from build123d import *

# Parameters (mm, degrees)
F0_W     = 203.2
F0_H     = 152.4
F1_DEPTH = 19.05
F2_SIZE  = 6.35
F4_D     = 25.4
F5_W     = 31.75
F5_H     = 31.75
F7_R     = 6.35
F8_SIZE  = 3.81


with BuildPart() as f1:
    # F0 (on Top) → F1 (new body)
    with BuildSketch(Plane.XY):
        Rectangle(F0_W, F0_H)
    extrude(amount=F1_DEPTH)

    # F2
    f2_edges = [f1.edges().sort_by_distance(p)[0] for p in [
        (0, -76.2, 19.05),
        (101.6, 0, 19.05),
        (-101.6, 0, 19.05),
        (0, 76.2, 19.05),
    ]]
    chamfer(f2_edges, length=F2_SIZE)

    # F4 (through all)
    with Locations(Plane.XY.offset(19.05)):
        with Locations((-69.85, 44.45), (69.85, 44.45), (69.85, -44.45), (-69.85, -44.45)):
            Hole(F4_D / 2)

    # F5 (on Front) → F6 (revolve)
    with BuildSketch(Plane.XZ):
        Polygon((0, 114.3), (0, 82.55), (31.75, 82.55), (44.45, 82.55), (44.45, 114.3), align=None)
        with Locations((15.875, 66.675)):
            Rectangle(F5_W, F5_H)
        Polygon((31.75, 50.8), (0, 50.8), (0, 19.05), (44.45, 19.05), (44.45, 50.8), align=None)
    revolve(axis=Axis((0, 0, 34.925), (0, 0, -1)))

    # F7
    f7_edges = [f1.edges().sort_by_distance(p)[0] for p in [
        (-44.45, 0, 114.3),
        (-44.45, 0, 19.05),
    ]]
    fillet(f7_edges, radius=F7_R)

    # F8
    f8_edges = [f1.edges().sort_by_distance(p)[0] for p in [
        (-44.45, 0, 50.8),
        (-44.45, 0, 82.55),
    ]]
    chamfer(f8_edges, length=F8_SIZE)


solid = f1.part
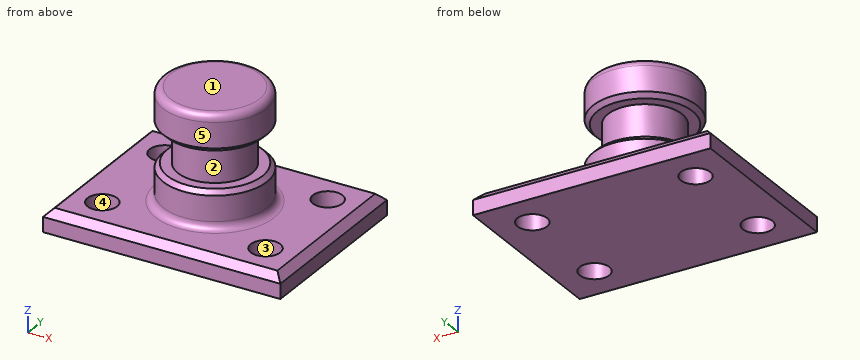
Input: part model. Units: mm. Frame: model coordinates. Face numbers are marked on the shaded views. A direction names the side the tool comes from. Give positions to 0.01 mm unless a question says otherwise; leave off trailing zeros. Loops run counter-clockwise (first coordinate to the right, second up) from the corner with the lowest first, then second, coordinate; pieces in that order, holes last. Notation, with made-up numbers: (7.5, -11) -> (33.5, -11) arc R11 cw to (33.5, 1) -> close; hole circle Ø10 at (77.25, 52.5). An arc over 180 degrees is marked (long way). Answer as a JSON object with one key per item and string values. Group by question number.
Item 1: Line query: probe 1 along X at (y, z) = (44, 10); probe 2 along Y at (x, z) = (-69, 10); probe 3 along Y at (x, z) = (64.5, 16.5). Output: solid intervals per line, ascending.
Item 2: Cut plane D-D, the plane z = 64.5. Return the cut outline in (x, y), and give its area (3 significant figures).
Item 3: Pull-direction query (Y, two-part tool) for the marked faces 1, 2 and 3; classes: released by +Y, released by -Y, zero draft, split by the parting line, or undercut.
Item 4: Pin query (flat end, axial travel): P1, Ø1, axis at x = 8, z = 78, coming from the -Y side; P2, Ø6, axis at x = 28, z = 87, coming from the -Y side; P3, Ø15, axis at x = -69.85, y = 44.45, coming from the +Z side; P4, Ø3, axis at y = -10, z = 21.5, coming from the +X side. Return the tip coordinate at first contact, or that it passes through.
Item 5: Cut plane B-B, the plane y = 0. Return the cut outline in (x, z).
Item 6: Cut plane C-C, the plane x = 0. Return the cut outline in (y, z), and give its area (3 significant figures).
Item 7: Reachability of the marked faces 4 and 5 from +Z, -Z, +X, -X, +Y, -Y: full face, straight path, thin tool, end or side. Return the list, or none.
Item 8: Cut plane A-A, the plane x = 78. Return the cut outline in (y, z).
Checks:
{
 "1": {"probe 1": "x = -101.6 to -82.54, -57.16 to 57.16, 82.54 to 101.6", "probe 2": "y = -76.2 to -57.12, -31.78 to 31.78, 57.12 to 76.2", "probe 3": "y = -72.4 to -55.97, -32.93 to 32.93, 55.97 to 72.4"},
 "2": {"outline": "circle Ø63.5 at (0, 0)", "area": "3,170 mm²"},
 "3": {"face 1": "zero draft", "face 2": "split by the parting line", "face 3": "undercut"},
 "4": {"P1": "stops at y = -30.85", "P2": "stops at y = -36.75", "P3": "passes through", "P4": "stops at x = 46.41"},
 "5": {"outline": "(-101.6, 0) -> (101.6, 0) -> (101.6, 12.7) -> (95.25, 19.05) -> (50.8, 19.05) arc R6.35 cw to (44.45, 25.4) -> (44.45, 46.99) -> (40.64, 50.8) -> (31.75, 50.8) -> (31.75, 82.55) -> (40.64, 82.55) -> (44.45, 86.36) -> (44.45, 107.95) arc R6.35 ccw to (38.1, 114.3) -> (-38.1, 114.3) arc R6.35 ccw to (-44.45, 107.95) -> (-44.45, 86.36) -> (-40.64, 82.55) -> (-31.75, 82.55) -> (-31.75, 50.8) -> (-40.64, 50.8) -> (-44.45, 46.99) -> (-44.45, 25.4) arc R6.35 cw to (-50.8, 19.05) -> (-95.25, 19.05) -> (-101.6, 12.7) -> close"},
 "6": {"outline": "(-76.2, 0) -> (76.2, 0) -> (76.2, 12.7) -> (69.85, 19.05) -> (50.8, 19.05) arc R6.35 cw to (44.45, 25.4) -> (44.45, 46.99) -> (40.64, 50.8) -> (31.75, 50.8) -> (31.75, 82.55) -> (40.64, 82.55) -> (44.45, 86.36) -> (44.45, 107.95) arc R6.35 ccw to (38.1, 114.3) -> (-38.1, 114.3) arc R6.35 ccw to (-44.45, 107.95) -> (-44.45, 86.36) -> (-40.64, 82.55) -> (-31.75, 82.55) -> (-31.75, 50.8) -> (-40.64, 50.8) -> (-44.45, 46.99) -> (-44.45, 25.4) arc R6.35 cw to (-50.8, 19.05) -> (-69.85, 19.05) -> (-76.2, 12.7) -> close", "area": "10,500 mm²"},
 "7": {"face 4": "+Z, -Z", "face 5": "+Z"},
 "8": {"outline": "(-76.2, 0) -> (-54.19, 0) -> (-54.19, 19.05) -> (-69.85, 19.05) -> (-76.2, 12.7) -> close; (-34.71, 0) -> (34.71, 0) -> (34.71, 19.05) -> (-34.71, 19.05) -> close; (54.19, 0) -> (76.2, 0) -> (76.2, 12.7) -> (69.85, 19.05) -> (54.19, 19.05) -> close"}
}
